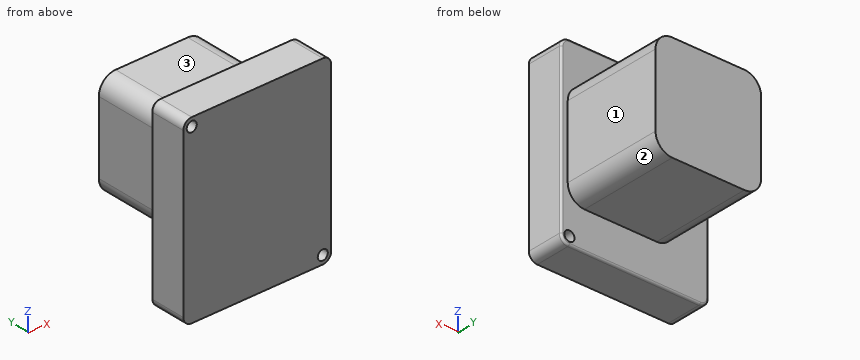
Autodesk Inventor part; units mm, degrees
ref_plane "YZ Plane" through (0, 0, 0) normal (1, 0, 0) x (0, 1, 0)
ref_plane "XZ Plane" through (0, 0, 0) normal (0, 1, 0) x (-1, 0, 0)
ref_plane "XY Plane" through (0, 0, 0) normal (0, 0, 1) x (1, 0, 0)
sketch "Sketch2" plane through (0, 0, 0) normal (0, 1, 0) x (-1, 0, 0)
  circle A0 centre (49.6189, -7.9375) radius 2.6988 construction
  circle A1 centre (0, -3.175) radius 2.6988 construction
  circle A2 centre (49.6189, -3.175) radius 1.905
  circle A3 centre (0, -65.405) radius 1.905
  arc A4 (49.6189, -68.58) -> (52.7939, -65.405) centre (49.6189, -65.405) ccw
  line L0 (52.7939, -65.405) -> (52.7939, -3.175)
  arc A5 (52.7939, -3.175) -> (49.6189, 0) centre (49.6189, -3.175) ccw
  line L1 (49.6189, 0) -> (0, 0)
  arc A6 (0, 0) -> (-3.175, -3.175) centre (0, -3.175) ccw
  line L2 (-3.175, -3.175) -> (-3.175, -65.405)
  arc A7 (-3.175, -65.405) -> (0, -68.58) centre (0, -65.405) ccw
  line L3 (0, -68.58) -> (49.6189, -68.58)
  circle A8 centre (49.6189, -65.405) radius 2.6988 construction
  circle A9 centre (0, -60.6425) radius 2.6988 construction
  point P0 (24.8095, -34.29)
extrude "Extrusion1" add sketch "Sketch2" along normal blind 13.97
fillet "Fillet1" radius 0.762 8 edges at (-52.7939, 13.97, -34.29) (-51.864, 13.97, -0.9299) (-24.8095, 13.97, 0) (2.2451, 13.97, -0.9299) (3.175, 13.97, -34.29) (2.2451, 13.97, -67.6501) (-24.8095, 13.97, -68.58) (-51.864, 13.97, -67.6501)
sketch "Sketch3" plane through (0, 13.97, 0) normal (0, 1, 0) x (1, 0, 0)
  line L0 (-52.0319, 3.175) -> (-52.0319, 65.405)
  line L1 (-39.37, 54.2925) -> (0.635, 54.2925)
  line L2 (0.635, 54.2925) -> (0.635, 14.2875)
  line L3 (0.635, 14.2875) -> (-39.37, 14.2875)
  line L4 (-39.37, 14.2875) -> (-39.37, 54.2925)
  line L5 (3.175, 3.175) -> (3.175, 65.405)
  point P0 (0, 0)
  point P1 (-52.0319, 34.29)
  point P2 (-39.37, 34.29)
  dimension "d3" = 40.005
  dimension "d4" = 40.005
  dimension "d5" = 2.54
extrude "Extrusion2" add sketch "Sketch3" along normal blind 38.1
fillet "Fillet2" radius 6.35 4 edges at (-39.37, 33.02, -14.2875) (0.635, 33.02, -14.2875) (0.635, 33.02, -54.2925) (-39.37, 33.02, -54.2925)
properties part number "Victor Controller" material "Nylon 6/6"
Input: part model. Units: mm. Frame: model coordinates. Face numbers are marked on the shaded views. A direction names the side the tool comes from. Give positions to 0.01 mm unless a question says otherwise; leave off trailing zeros. Order: outer loops, then holes, each group sorted by start corner. A loop starts at its lowest first (then second) coordinate and runs counter-clockwise, first axis right, second up. Notation, with made-up numbers: (42, 50.5) - (63, 50.5) arc R24 cw to (63, 65.5) - close; hole circle Ø5 at (2.5, 32). An arc over 180 degrees is marked (long way). Answer as a JSON object with one key per item and string values. Group by question number.
Q1. Cut plane A-A, the plane x = -19.5. Output: boundary loops of the cut face in (y, z).
Q2. Line query: probe 1 along Z at (x, y) = (0, 5.25); probe 2 along X at (y, z) = (48, -45.5) (3 decimals); probe 3 along Z at (x, y) = (-19.5, 38). Output: solid intervals per line, ascending.
Q3. First-contact query: pin 1 Ø13.5 at (y, z) = (42, -40.5) entering from -X; pin 2 Ø5 at (x, z) = (0, -65.405) entering from +Y; pin 3 Ø6 at (y, z) = (39.5, -50) entering from +X (3 decimals). Flat tips, straight axial feed; report the tip coordinate or a pass-through.
Q4. Set-up query: the marked faces 1, 2 and 3. Return all of +Z, -Z, +X, -X, +Y, -Y with unobstructed straight access to the full face (end or side cutting, diameter ignored); none if empty.
Q5. Cut plane C-C, the plane z = -53. Output: boundary loops of the cut face in (x, y) (3 decimals), then the cut area to 3 significant figures.
Results:
{
 "1": {"outline": "(0, -68.58) - (13.21, -68.58) arc R0.76 ccw to (13.97, -67.82) - (13.97, -54.29) - (52.07, -54.29) - (52.07, -14.29) - (13.97, -14.29) - (13.97, -0.76) arc R0.76 ccw to (13.21, 0) - (0, 0) - close"},
 "2": {"probe 1": "-68.58 to -67.31, -63.5 to 0", "probe 2": "-39.37 to 0.635", "probe 3": "-54.29 to -14.29"},
 "3": {"pin 1": "x = -39.37", "pin 2": "y = 13.97", "pin 3": "x = 0.635"},
 "4": {"face 1": "+Z, -Z, +X, +Y", "face 2": "-Z, +X, +Y", "face 3": "+Z, +X, -X, +Y"},
 "5": {"outline": "(-52.794, 0) - (3.175, 0) - (3.175, 13.208) arc R0.762 ccw to (2.413, 13.97) - (-1.875, 13.97) - (-1.875, 52.07) - (-36.86, 52.07) - (-36.86, 13.97) - (-52.032, 13.97) arc R0.762 ccw to (-52.794, 13.208) - close", "area": "2,110 mm^2"}
}
